```python
from build123d import *

# Parameters (mm, degrees)
SKETCH1_R                      = 2
SKETCH1_R_2                    = 3.125
SKETCH1_R_3                    = 1.7
BOSS_EXTRUDE1_DEPTH            = 10
FILLET2_R                      = 5
FILLET1_R                      = 2
SKETCH1_4_R                    = 3.125
CUT_EXTRUDE3_DEPTH             = 5.07
SKETCH1_7_R                    = 1.7
CUT_EXTRUDE6_DEPTH             = 10
CUT_EXTRUDE5_DEPTH             = 3
SKETCH1_5_R                    = 2
CUT_EXTRUDE4_DEPTH             = 2.48
SKETCH4_R                      = 1.5
CUT_EXTRUDE7_DEPTH             = 10
SKETCH5_R                      = 2.725
CUT_EXTRUDE8_DEPTH             = 2.8
BOSS_EXTRUDE2_DEPTH            = 10
BOSS_EXTRUDE3_DEPTH            = 35
FILLET13_R                     = 5
SKETCH10_W                     = 8
SKETCH10_H                     = 6
CUT_EXTRUDE12_DEPTH            = 40
FILLET14_R                     = 2
SKETCH27_W                     = 50.098907978
SKETCH27_H                     = 10
CUT_EXTRUDE22_DEPTH            = 35
FILLET17_R                     = 3
CBORE_FOR_M3_SHCS1_D           = 3.4
CBORE_FOR_M3_SHCS1_DEPTH       = 20
CBORE_FOR_M3_SHCS1_CBORE_D     = 6.5
CBORE_FOR_M3_SHCS1_CBORE_DEPTH = 3
CBORE_FOR_M3_SHCS1_TIP         = 1.021463052


with BuildPart() as part:
    # Sketch1 → Boss-Extrude1 (new body)
    with BuildSketch(Plane(origin=(0, 0, 0), x_dir=(1, 0, 0), z_dir=(0, 1, 0))):
        with BuildLine():
            ThreePointArc((-11.409245094, 8.977987014), (-9.849239736, 9.28), (-8.289234378, 8.977987014))
            ThreePointArc((-8.289234378, 8.977987014), (-5.835653376, 8.254222737), (-3.289234378, 8.01))
            Line((-3.289234378, 8.01), (38.12, 8.01))
            Line((38.12, 8.01), (38.12, -3.81))
            Line((38.12, -3.81), (28.478275237, -3.81))
            Line((28.478275237, -3.81), (26.178275237, 0))
            Line((26.178275237, 0), (-26.178275237, 0))
            Line((-26.178275237, 0), (-28.478275237, -3.81))
            Line((-28.478275237, -3.81), (-38.12, -3.81))
            Line((-38.12, -3.81), (-38.12, 8.01))
            Line((-38.12, 8.01), (-16.409245094, 8.01))
            ThreePointArc((-16.409245094, 8.01), (-13.862826096, 8.254222737), (-11.409245094, 8.977987014))
        make_face()
        with Locations((22, 4.005)):
            Circle(SKETCH1_R, mode=Mode.SUBTRACT)
        with Locations((-22, 4.005)):
            Circle(SKETCH1_R, mode=Mode.SUBTRACT)
        with Locations((-32.12, 1.98)):
            Circle(SKETCH1_R_2, mode=Mode.SUBTRACT)
        with Locations((32.12, 1.98)):
            Circle(SKETCH1_R_2, mode=Mode.SUBTRACT)
        with Locations((-9.849239736, 5.1)):
            Circle(SKETCH1_R_3, mode=Mode.SUBTRACT)
        with BuildLine():
            ThreePointArc((11.912105026, 2.53), (14.127105026, 4.745), (11.912105026, 6.96))
            Line((11.912105026, 6.96), (5.992105026, 6.96))
            ThreePointArc((5.992105026, 6.96), (3.777105026, 4.745), (5.992105026, 2.53))
            Line((5.992105026, 2.53), (11.912105026, 2.53))
        make_face(mode=Mode.SUBTRACT)
        with Locations((-22, 4.005)):
            Circle(SKETCH1_R)
        with Locations((-9.849239736, 5.1)):
            Circle(SKETCH1_R_3)
        with Locations((-32.12, 1.98)):
            Circle(SKETCH1_R_2)
        with BuildLine():
            Line((5.992105026, 2.53), (11.912105026, 2.53))
            ThreePointArc((11.912105026, 2.53), (14.127105026, 4.745), (11.912105026, 6.96))
            Line((11.912105026, 6.96), (5.992105026, 6.96))
            ThreePointArc((5.992105026, 6.96), (3.777105026, 4.745), (5.992105026, 2.53))
        make_face()
        with Locations((22, 4.005)):
            Circle(SKETCH1_R)
        with Locations((32.12, 1.98)):
            Circle(SKETCH1_R_2)
    extrude(amount=-BOSS_EXTRUDE1_DEPTH)

    # Fillet2
    fillet2_edges = [part.edges().sort_by_distance(p)[0] for p in [
        (28.478275237, -5, 3.81),
        (-28.478275237, -5, 3.81),
    ]]
    fillet(fillet2_edges, radius=FILLET2_R)

    # Fillet1
    fillet1_edges = [part.edges().sort_by_distance(p)[0] for p in [
        (26.178275237, -5, 0),
        (-26.178275237, -5, 0),
    ]]
    fillet(fillet1_edges, radius=FILLET1_R)

    # Sketch1_4 → Cut-Extrude3 (cut)
    with BuildSketch(Plane(origin=(0, 0, 0), x_dir=(1, 0, 0), z_dir=(0, 1, 0))):
        with Locations(Location((32.12, 1.98, 0), (0, 0, 270))):
            Circle(SKETCH1_4_R)
        with Locations(Location((-32.12, 1.98, 0), (0, 0, 270))):
            Circle(SKETCH1_4_R)
    extrude(amount=-CUT_EXTRUDE3_DEPTH, mode=Mode.SUBTRACT)

    # Sketch1_7 → Cut-Extrude6 (cut)
    with BuildSketch(Plane(origin=(0, 0, 0), x_dir=(1, 0, 0), z_dir=(0, 1, 0))):
        with Locations(Location((-9.849239736, 5.1, 0), (0, 0, 270))):
            Circle(SKETCH1_7_R)
    extrude(amount=-CUT_EXTRUDE6_DEPTH, mode=Mode.SUBTRACT)

    # Sketch1_6 → Cut-Extrude5 (cut)
    with BuildSketch(Plane(origin=(0, 0, 0), x_dir=(1, 0, 0), z_dir=(0, 1, 0))):
        with BuildLine():
            Line((5.992105026, 2.53), (11.912105026, 2.53))
            ThreePointArc((11.912105026, 2.53), (14.127105026, 4.745), (11.912105026, 6.96))
            Line((11.912105026, 6.96), (5.992105026, 6.96))
            ThreePointArc((5.992105026, 6.96), (3.777105026, 4.745), (5.992105026, 2.53))
        make_face()
    extrude(amount=-CUT_EXTRUDE5_DEPTH, mode=Mode.SUBTRACT)

    # Sketch1_5 → Cut-Extrude4 (cut)
    with BuildSketch(Plane(origin=(0, 0, 0), x_dir=(1, 0, 0), z_dir=(0, 1, 0))):
        with Locations(Location((-22, 4.005, 0), (0, 0, 270))):
            Circle(SKETCH1_5_R)
        with Locations(Location((22, 4.005, 0), (0, 0, 270))):
            Circle(SKETCH1_5_R)
    extrude(amount=-CUT_EXTRUDE4_DEPTH, mode=Mode.SUBTRACT)

    # Sketch4 → Cut-Extrude7 (cut)
    with BuildSketch(Plane(origin=(0, 0, 0), x_dir=(1, 0, 0), z_dir=(0, 1, 0))):
        with Locations(Location((-22, 4.005, 0), (0, 0, 270))):
            Circle(SKETCH4_R)
        with Locations(Location((22, 4.005, 0), (0, 0, 270))):
            Circle(SKETCH4_R)
    extrude(amount=-CUT_EXTRUDE7_DEPTH, mode=Mode.SUBTRACT)

    # Sketch5 → Cut-Extrude8 (cut)
    with BuildSketch(Plane.XZ.offset(10)):
        with Locations(Location((22, -4.005, 0), (0, 0, 270))):
            Circle(SKETCH5_R)
        with Locations(Location((-22, -4.005, 0), (0, 0, 90))):
            Circle(SKETCH5_R)
    extrude(amount=-CUT_EXTRUDE8_DEPTH, mode=Mode.SUBTRACT)

    # Sketch6 → Boss-Extrude2 (add)
    with BuildSketch(Plane(origin=(0, 0, 0), x_dir=(1, 0, 0), z_dir=(0, 1, 0))):
        with BuildLine():
            Line((-38.12, 8.01), (-38.12, 18.01))
            Line((-38.12, 18.01), (38.12, 18.01))
            Line((38.12, 18.01), (38.12, 8.01))
            Line((38.12, 8.01), (-3.289234378, 8.01))
            ThreePointArc((-3.289234378, 8.01), (-5.835653376, 8.254222737), (-8.289234378, 8.977987014))
            ThreePointArc((-8.289234378, 8.977987014), (-9.849239736, 9.28), (-11.409245094, 8.977987014))
            ThreePointArc((-11.409245094, 8.977987014), (-13.862826096, 8.254222737), (-16.409245094, 8.01))
            Line((-16.409245094, 8.01), (-38.12, 8.01))
        make_face()
    extrude(amount=-BOSS_EXTRUDE2_DEPTH)

    # Sketch8 → Boss-Extrude3 (add)
    with BuildSketch(Plane.XZ.offset(10)):
        with BuildLine():
            Line((18.950546011, 0), (-18.950546011, 0))
            Line((-18.950546011, 0), (-18.950546011, -4.005))
            ThreePointArc((-18.950546011, -4.005), (-22, -7.054453989), (-25.049453989, -4.005))
            Line((-25.049453989, -4.005), (-25.049453989, 0))
            ThreePointArc((-25.049453989, 0), (-26.032503369, 0.25827272), (-26.761657912, 0.966386084))
            Line((-26.761657912, 0.966386084), (-27.019818549, 1.394034791))
            ThreePointArc((-27.019818549, 1.394034791), (-28.842704905, 3.164318199), (-31.300328355, 3.81))
            Line((-31.300328355, 3.81), (-38.12, 3.81))
            Line((-38.12, 3.81), (-38.12, -18.01))
            Line((-38.12, -18.01), (38.12, -18.01))
            Line((38.12, -18.01), (38.12, 3.81))
            Line((38.12, 3.81), (31.300328355, 3.81))
            ThreePointArc((31.300328355, 3.81), (28.842704905, 3.164318199), (27.019818549, 1.394034791))
            Line((27.019818549, 1.394034791), (26.761657912, 0.966386084))
            ThreePointArc((26.761657912, 0.966386084), (26.032503369, 0.25827272), (25.049453989, 0))
            Line((25.049453989, 0), (25.049453989, -4.005))
            ThreePointArc((25.049453989, -4.005), (22, -7.054453989), (18.950546011, -4.005))
            Line((18.950546011, -4.005), (18.950546011, 0))
        make_face()
    extrude(amount=BOSS_EXTRUDE3_DEPTH)

    # Fillet13
    fillet13_edges = [part.edges().sort_by_distance(p)[0] for p in [
        (-38.12, -22.5, -18.01),
    ]]
    fillet(fillet13_edges, radius=FILLET13_R)

    # Sketch10 → Cut-Extrude12 (cut)
    with BuildSketch(Plane(origin=(38.12, 0, 0), x_dir=(0, 0, -1), z_dir=(1, 0, 0))):
        with Locations((12.01, -3)):
            Rectangle(SKETCH10_W, SKETCH10_H)
    extrude(amount=-CUT_EXTRUDE12_DEPTH, mode=Mode.SUBTRACT)

    # Fillet14
    fillet14_edges = [part.edges().sort_by_distance(p)[0] for p in [
        (-1.88, -3, -16.01),
        (18.12, -6, -16.01),
        (-1.88, -3, -8.01),
    ]]
    fillet(fillet14_edges, radius=FILLET14_R)

    # Sketch27 → Cut-Extrude22 (cut)
    with BuildSketch(Plane.XZ.offset(45)):
        with Locations((0, -5)):
            Rectangle(SKETCH27_W, SKETCH27_H)
    extrude(amount=-CUT_EXTRUDE22_DEPTH, mode=Mode.SUBTRACT)

    # Fillet17
    fillet17_edges = [part.edges().sort_by_distance(p)[0] for p in [
        (-25.049453989, -27.5, -10),
        (25.049453989, -27.5, -10),
    ]]
    fillet(fillet17_edges, radius=FILLET17_R)

    # CBORE for M3 SHCS1
    with Locations(Plane(origin=(0, -53, 22.49), x_dir=(-1, 0, 0), z_dir=(0, -1, 0))):
        with Locations((-5, 36.495), (5, 36.495)):
            CounterBoreHole(CBORE_FOR_M3_SHCS1_D / 2, CBORE_FOR_M3_SHCS1_CBORE_D / 2, CBORE_FOR_M3_SHCS1_CBORE_DEPTH, depth=CBORE_FOR_M3_SHCS1_DEPTH)
            with Locations((0, 0, -(CBORE_FOR_M3_SHCS1_DEPTH + CBORE_FOR_M3_SHCS1_TIP / 2))):  # 118° drill point
                Cone(0, CBORE_FOR_M3_SHCS1_D / 2, CBORE_FOR_M3_SHCS1_TIP, mode=Mode.SUBTRACT)


solid = part.part
```
Input: part model. Units: mm. Frame: model coordinates. A direction names the side the tool comes from. Give positions to 0.01 mm unless a question says otherwise; leave off trailing zeros. Loops run counter-clockwise (first coordinate to the right, second up) from the corner with the lowest first, then second, coordinate; pieces in that order, holes last. Notation, with made-up numbers: (84, 81.5) -> (122, 81.5) arc R19 ccw to (122, 115.5) -> close; hole circle Ø9 at (-29, 82.5). An arc over 180 degrees is marked (long way). Use a Markdown table: item, result.
Q1. Section query C-C, the plane z = -11.25. Return the cut outline in (x, y), plus the area to 3 significant figures.
Entries:
| item | result |
|---|---|
| outline | (-38.12, -45) -> (38.12, -45) -> (38.12, -6) -> (-1.88, -6) -> (-1.88, 0) -> (-38.12, 0) -> close |
| area | 3,190 mm² |
Q2. Section query B-B, the plane x = 17. Return the cut outline in (y, z), plus the area to 3 significant figures.
Entries:
| item | result |
|---|---|
| outline | (-45, -18.01) -> (0, -18.01) -> (0, -16.01) -> (-4, -16.01) arc R2 cw to (-6, -14.01) -> (-6, -8.01) -> (0, -8.01) -> (0, 0) -> (-10, 0) -> (-10, -10) -> (-45, -10) -> close |
| area | 413 mm² |
Q3. First-contact query: P1, Ø5, axis at x = 22, z = -4.005, coming from the -Y side; P2, Ø8, axis at x = 6.5, z = -5, coming from the -Y side; P3, Ø1.5, axis at x = 7.5, y = -1, coming from the +Z side. Flat tips, straight axial feed; report the tip coordinate or a pass-through.
Entries:
| item | result |
|---|---|
| P1 | stops at y = -7.2 |
| P2 | stops at y = -10 |
| P3 | stops at z = 0 |
Q4. Access query for faces 4 (the flat face through (-1.88, -3, -12)), 5 (the cylindrical face through (24.19, -27.26, -9.1)), 6 (the flat face through (20.8, -7.2, -5.2)), 7 (the flat face through (0, -5, 0)), 8 (the cylindrical face through (3.778, -1.479, -4.794)). Directions: +Z, -Z, +X, -X, +Y, -Y. A direction counts if a zero-diameter tool reaches every point of the face in a straight line with its end or side. Return the directions, or none.
Entries:
| item | result |
|---|---|
| face 4 | +X, +Y |
| face 5 | +Z, -Y |
| face 6 | -Y |
| face 7 | +Z, +Y, -Y |
| face 8 | +Y |
Q5. Section query A-A, the plane y = -27.5. Return the cut outline in (x, z), plus the area to 3 significant figures.
Entries:
| item | result |
|---|---|
| outline | (-38.12, -13.01) arc R5 ccw to (-33.12, -18.01) -> (38.12, -18.01) -> (38.12, 3.81) -> (31.3, 3.81) arc R5 ccw to (27.02, 1.39) -> (26.76, 0.97) arc R2 cw to (25.05, 0) -> (25.05, -7) arc R3 cw to (22.05, -10) -> (-22.05, -10) arc R3 cw to (-25.05, -7) -> (-25.05, 0) arc R2 cw to (-26.76, 0.97) -> (-27.02, 1.39) arc R5 ccw to (-31.3, 3.81) -> (-38.12, 3.81) -> close |
| area | 951 mm² |
Q6. Ray query, probe 1 along X at (y, z) = (-23, -0.5); probe 2 along X at (y, z) = (-18.5, 3.25); probe 3 along Z at (x, y) = (-5, -41) (3 decimals). Return the intervals inside material, ascending. Write a range as from..to.
Entries:
| item | result |
|---|---|
| probe 1 | x = -38.12..-25.05, 25.05..38.12 |
| probe 2 | x = -38.12..-29, 29..38.12 |
| probe 3 | z = -18.01..-15.705, -12.305..-10 |
Q7. Section query D-D, the plane y = -39.5. Return the cut outline in (x, z) (3 decimals).
Entries:
| item | result |
|---|---|
| outline | (-38.12, -13.01) arc R5 ccw to (-33.12, -18.01) -> (38.12, -18.01) -> (38.12, 3.81) -> (31.3, 3.81) arc R5 ccw to (27.02, 1.394) -> (26.762, 0.966) arc R2 cw to (25.049, 0) -> (25.049, -7) arc R3 cw to (22.049, -10) -> (-22.049, -10) arc R3 cw to (-25.049, -7) -> (-25.049, 0) arc R2 cw to (-26.762, 0.966) -> (-27.02, 1.394) arc R5 ccw to (-31.3, 3.81) -> (-38.12, 3.81) -> close; hole circle Ø3.4 at (-5, -14.005); hole circle Ø3.4 at (5, -14.005) |
Q8. Pull-direction query (X, two-part tool) for faces 1 (the flat face through (19, -2, -16.01)), 2 (the cylindrical face through (23.487, -4.807, -4.2)), 3 (the flat face through (38.12, -22, -7)); classes: pulls with the +X half, pulls with the -X half, needs draft (parallel to the pull), parting line crosses it, or undercut.
Entries:
| item | result |
|---|---|
| face 1 | needs draft |
| face 2 | undercut |
| face 3 | pulls with the +X half |
